Part model, mm, in its own coordinate system. A direction names the side the tool comes from. Give positions to 0.01 mm unless a question says otherwise; leave off trailing zeros. Loops run counter-clockwise (first coordinate to the right, second up) from the corner with the lowest first, then second, coordinate; pieces in that order, holes last. Notation, with made-up numbers: (61.5, 86.5) -> (89.5, 86.5) arc R15 ccw to (89.5, 100.5) -> close; hole circle Ø10 at (29, 4). An arc over 180 degrees is marked (long way). Write item = value, one per line.
from build123d import *

# Parameters (mm, degrees)
F0_R     = 39.6875
F1_DEPTH = 25.4
F2_R     = 44.45
F3_DEPTH = 4.7625
F4_R     = 44.551262
F4_R_2   = 39.6875
F5_DEPTH = 4.7625


with BuildPart() as f1:
    # F0 (on Front) → F1 (new body)
    with BuildSketch(Plane.XZ):
        Polygon((31.162481, 53.975), (-31.162481, 53.975), (-62.324962, 0), (-31.162481, -53.975), (31.162481, -53.975), (62.324962, 0), align=None)
        Circle(F0_R, mode=Mode.SUBTRACT)
    extrude(amount=F1_DEPTH)

    # F2 (on Front) → F3 (cut)
    with BuildSketch(Plane.XZ):
        Circle(F2_R)
    extrude(amount=F3_DEPTH, mode=Mode.SUBTRACT)

    # F4 (on face) → F5 (cut)
    with BuildSketch(Plane.XZ.offset(25.4)):
        Circle(F4_R)
        Circle(F4_R_2, mode=Mode.SUBTRACT)
    extrude(amount=-F5_DEPTH, mode=Mode.SUBTRACT)


solid = f1.part
1) Pull direction X, two halves, no side cores. Call faces 1 (the face through (-46.96, -12.52, -26.61)), 2 (the face through (9, -25.4, -44)), 3 (the face through (42.397, -2.348, 13.352)): pulls with the +X half, pulls with the -X half, needs draft (parallel to the pull), parting line crosses it, or undercut.
Resolved:
face_1 = pulls with the -X half
face_2 = needs draft
face_3 = undercut
2) Slice it at A-A, the plane y = -12. List the corners of the cut face in (x, z) (1 decimal), and give its area (3 significant figures).
Resolved:
outline = (-62.3, 0) -> (-31.2, -54) -> (31.2, -54) -> (62.3, 0) -> (31.2, 54) -> (-31.2, 54) -> close; hole circle Ø79.4 at (0, 0)
area = 5,140 mm²
3) Drop flat-ended pins along their axis: P1, Ø12, axis at x = -23, z = 29, coming from the -Y side; P2, Ø3, axis at x = -42.5, y = -18, coming from the +Z side; P3, Ø1.5, axis at x = 49.5, y = -8.5, coming from the +Z side. Give the stop position or say it passes through.
Resolved:
P1 = -20.64
P2 = 36.94
P3 = 23.51
4) Which spindle directions (+Z, -Z, +X, -X, +Y, -Y) get a long thin tool onto all of the face, cutting with end or side? Do faces 4 (the face through (-40, -20.638, -3)), 5 (the face through (46.96, -12.52, 26.61)), 6 (the face through (-16.7, -4.762, 36.4)). Say none if no direction does.
Resolved:
face_4 = -Y
face_5 = +Z, +X, +Y, -Y
face_6 = +Y
5) Drill centre lines: line 1 along Z through (x, y) = (0, -23.1) (3 decimals); line 2 along Z through (x, y) = (0, -13) (1 decimal); line 3 along X through (y, z) = (-14, 0). Where is each one in solid material? Low to high. Write a range as [from, to].
Resolved:
line_1 = [-53.975, -44.551], [44.551, 53.975]
line_2 = [-54, -39.7], [39.7, 54]
line_3 = [-62.32, -39.69], [39.69, 62.32]
6) Slice it at C-C, the plane z = -15. List the corners of the cut face in (x, y).
Resolved:
outline = (-53.66, -25.4) -> (-41.95, -25.4) -> (-41.95, -20.64) -> (-36.74, -20.64) -> (-36.74, -4.76) -> (-41.84, -4.76) -> (-41.84, 0) -> (-53.66, 0) -> close; (36.74, -20.64) -> (41.95, -20.64) -> (41.95, -25.4) -> (53.66, -25.4) -> (53.66, 0) -> (41.84, 0) -> (41.84, -4.76) -> (36.74, -4.76) -> close
